Work out the finished part from the listing and answer in its coordinate system (mm). Face numbers are marked on the shaded views. A direction names the side the tool comes from. Give positions to 0.01 mm unless a question says otherwise; leave off trailing zeros. Order: outer loops, then holes, each group sorted by start corner. A loop starts at its lowest first (then second) coordinate and runs counter-clockwise, first axis right, second up. Notation, with made-up numbers: (63.25, 87.25) -> (78.25, 87.25) arc R28 ccw to (78.25, 109.25) -> close; hole circle Ø2 at (25.5, 78). An arc over 180 degrees is marked (long way). Use a Markdown table: item, result. Add a question column.
```python
from build123d import *

# Parameters (mm, degrees)
F1_DEPTH = 7.62
F3_DEPTH = 25.4


# Not quite as in the source:
# - ends of sketch curves that miss each other by under 0.0002 mm in the source are joined


with BuildPart() as f1:
    # F0 (on Top) → F1 (new body)
    with BuildSketch(Plane.XY):
        Polygon((0, 56.5666313121), (-12.7, 17.48005039), (12.7, 17.48005039), align=None)
        Polygon((12.7, 17.48005039), (-12.7, 17.48005039), (-20.5490316571, -6.6767851239), (0, -21.6065305321), (20.5490316571, -6.6767851239), align=None)
        Polygon((-20.5490316571, -6.6767851239), (-12.7, 17.48005039), (-53.7980635454, 17.48005039), align=None)
        Polygon((53.7980636, 17.48005039), (12.7, 17.48005039), (20.5490316571, -6.6767851239), align=None)
        Polygon((0, -21.6065305321), (-20.5490316571, -6.6767851239), (-33.2490320312, -45.7633663178), align=None)
        Polygon((33.2490317454, -45.7633663178), (20.5490316571, -6.6767851239), (0, -21.6065305321), align=None)
    extrude(amount=F1_DEPTH)

    # F2 (on Top) → F3 (cut)
    with BuildSketch(Plane.XY):
        Polygon((23.131839931, 17.1561446041), (7.3025235906, 34.8562002182), (-13.5633936152, 2.1902460139), (4.1366601363, 5.3561092354), (-8.3828903735, -21.1220216006), (23.131839931, 12.2634470463), (2.4098258, 9.5292925835), align=None)
    extrude(amount=F3_DEPTH, mode=Mode.SUBTRACT)


solid = f1.part
```
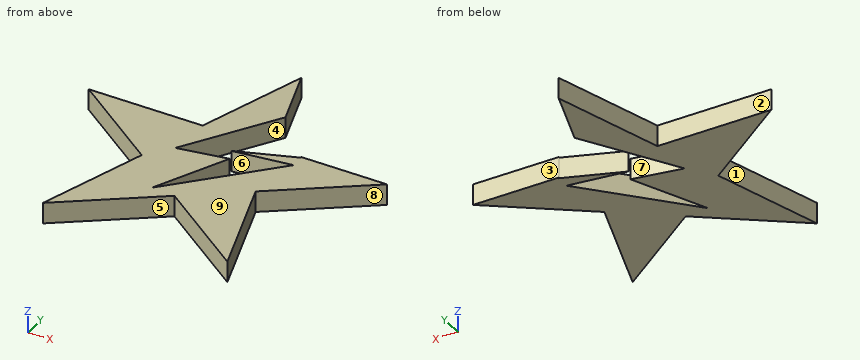
1) The part is cut by section C-C, the plane x = -4.5. Determine the outline of the cut face in (y, z), then the cut area to 3 significant figures.
2) The part is cut by section D-D, the plane x = 15. Determine the outline of the cut face in (y, z), then the cut area to 3 significant figures.
3) Determine the mould class of the marked faces 6, 7, 8 and 9 for opening direction X: released by +X, released by -X, zero draft, split by the parting line, or undercut.
4) Which of the six approach directions +Z, -Z, +X, -X, +Y, -Y give full straight-line access (tool end or side, diameter ignored) to the marked faces 1, 2, 3, 4 and 5?
5) Straight lines are drawn through the part: line 1 (X direction, y = -13, z = 3.5); line 2 (X direction, y = -27, z = 5); line 3 (Y direction, x = 20.5, z = 7). For each, find the intervals that lie inside material, in ascending order.
6) The part is cut by section B-B, the plane y = -15. Determine the outline of the cut face in (x, z).
7) Flat-ended cylindrical pins translate along their axes: pin 1 (2 mm diameter, centred on y = -10, z = 6.5, fed in from -X); pin 2 (1 mm diameter, centred on y = 33, z = 2.5, fed in from +X); pin 3 (3 mm diameter, centred on y = 10, z = 4.5, fed in from +X). Find the tip coordinate at first contact, or state that the pin passes through.
8) The part is cut by section A-A, the plane z = 6. Determine the outline of the cut face in (x, y).
A:
| question | item | result |
|---|---|---|
| 1 | outline | (-24.88, 0) -> (-17.01, 0) -> (-17.01, 7.62) -> (-24.88, 7.62) -> close; (-12.91, 0) -> (3.81, 0) -> (3.81, 7.62) -> (-12.91, 7.62) -> close; (16.38, 0) -> (42.72, 0) -> (42.72, 7.62) -> (16.38, 7.62) -> close |
| 1 | area | 388 mm^2 |
| 2 | outline | (-32.5, 0) -> (3.65, 0) -> (3.65, 7.62) -> (-32.5, 7.62) -> close; (11.19, 0) -> (14.16, 0) -> (14.16, 7.62) -> (11.19, 7.62) -> close |
| 2 | area | 298 mm^2 |
| 3 | face 6 | undercut |
| 3 | face 7 | undercut |
| 3 | face 8 | released by +X |
| 3 | face 9 | zero draft |
| 4 | face 1 | +Z, -Z, -X |
| 4 | face 2 | +Z, -Z, -X, +Y |
| 4 | face 3 | +Z, -Z, +X, +Y |
| 4 | face 4 | +Z, -Z |
| 4 | face 5 | +Z, -Z, -Y |
| 5 | line 1 | -22.6 to -4.54, -0.72 to 22.6 |
| 5 | line 2 | -27.15 to -7.42, 7.42 to 27.15 |
| 5 | line 3 | -36.5 to 9.48, 11.92 to 16.19 |
| 6 | outline | (-23.25, 0) -> (-5.49, 0) -> (-5.49, 7.62) -> (-23.25, 7.62) -> close; (-2.6, 0) -> (23.25, 0) -> (23.25, 7.62) -> (-2.6, 7.62) -> close |
| 7 | pin 1 | x = -21.95 |
| 7 | pin 2 | x = 6.44 |
| 7 | pin 3 | x = 45.57 |
| 8 | outline | (-53.8, 17.48) -> (-20.55, -6.68) -> (-33.25, -45.76) -> (0, -21.61) -> (33.25, -45.76) -> (20.55, -6.68) -> (53.8, 17.48) -> (22.84, 17.48) -> (23.13, 17.16) -> (2.41, 9.53) -> (23.13, 12.26) -> (-8.38, -21.12) -> (4.14, 5.36) -> (-13.56, 2.19) -> (7.14, 34.6) -> (0, 56.57) -> (-12.7, 17.48) -> close |
